Autodesk Inventor part; units mm, degrees
ref_plane "YZ Plane" through (0, 0, 0) normal (1, 0, 0) x (0, 1, 0)
ref_plane "XZ Plane" through (0, 0, 0) normal (0, 1, 0) x (-1, 0, 0)
ref_plane "XY Plane" through (0, 0, 0) normal (0, 0, 1) x (1, 0, 0)
sketch "Sketch1" plane through (0, 0, 0) normal (0, 0, 1) x (1, 0, 0)
  line L0 (-112.5, -225) -> (112.5, -225)
  line L1 (112.5, -225) -> (112.5, 225)
  line L2 (112.5, 225) -> (-112.5, 225)
  line L3 (-112.5, 225) -> (-112.5, -225)
  line L4 (-112.5, -225) -> (112.5, 225) construction
  line L5 (112.5, -225) -> (-112.5, 225) construction
  point P0 (0, 0)
  dimension "d0" = 225
  dimension "d1" = 450
extrude "Extrusion1" add sketch "Sketch1" along normal blind 4
sketch "Sketch2" plane through (0, 0, 4) normal (0, 0, 1) x (1, 0, 0)
  line L0 (-112.5, 225) -> (12.5, 225)
  line L1 (12.5, 225) -> (-112.5, -50)
  line L2 (-112.5, 225) -> (-112.5, -50)
  line L3 (112.5, -225) -> (112.5, 225)
  line L4 (112.5, -50) -> (112.5, 225)
  line L5 (112.5, 225) -> (62.5, 225)
  line L6 (-112.5, -225) -> (112.5, -225)
  line L7 (-112.5, -50) -> (-112.5, 225)
  line L8 (-112.5, 225) -> (12.5, 225)
  point P0 (0, 0)
  dimension "d8" = 175
extrude "Extrusion2" cut sketch "Sketch2" against normal blind 4
properties part number "SidePanel"
Model file for the job. Use its own axes, mm. Give positions to 0.01 mm unless a question says otherwise; leave off trailing zeros. Loops run counter-clockwise (first coordinate to the right, second up) from the corner with the lowest first, then second, coordinate; pieces in that order, holes last. Notation, with made-up numbers: (-3, 25.5) - (12, 25.5) arc R21 ccw to (12, 35.5) - close; hole circle Ø11 at (-39.5, -35.5). An arc over 180 degrees is marked (long way). Use one line per item in the form item = value.
(1) Drill centre lines: L1, parallel to Y at x = -100, z = 2.15; L2, parallel to X at y = 15, z = 1.35; L3, parallel to X at y = 203, z = 1.35. Where is each one in solid material? Low to high.
Determined:
L1 = -225 to -22.5
L2 = -82.95 to 112.5
L3 = 2.5 to 112.5
(2) Cut at B-B (z = 2.85). Give the cut face in (x, y), then the cut area to 3 significant figures.
Determined:
outline = (-112.5, -225) - (112.5, -225) - (112.5, 225) - (12.5, 225) - (-112.5, -50) - close
area = 84,100 mm^2
(3) Cut at A-A (x = -52). Give the cut face in (y, z), then the cut area to 3 significant figures.
Determined:
outline = (-225, 0) - (83.1, 0) - (83.1, 4) - (-225, 4) - close
area = 1,230 mm^2
(4) Cut at C-C (y = -8). Give the cut face in (x, z).
Determined:
outline = (-93.41, 0) - (112.5, 0) - (112.5, 4) - (-93.41, 4) - close
